from build123d import *

# Parameters (mm, degrees)
F0_W     = 127
F0_H     = 76.2
F1_DEPTH = 50.8
F2_T     = -2.54
F4_DEPTH = 76.2


with BuildPart() as f1:
    # F0 (on Top) → F1 (new body)
    with BuildSketch(Plane.XY):
        with Locations((63.5, 38.1)):
            Rectangle(F0_W, F0_H)
    extrude(amount=F1_DEPTH)

    # F2
    f2_openings = [f1.faces().sort_by_distance(p)[0] for p in [
        (63.5, 38.1, 50.8),
    ]]
    offset(amount=F2_T, openings=f2_openings)

    # F3 (on face) → F4 (join)
    with BuildSketch(Plane.XZ):
        Polygon((50.8, 50.8), (0, 0), (51.892955, 0), align=None)
    extrude(amount=F4_DEPTH)


solid = f1.part
CAD build for the part. Positions are in the model's coordinates, mm. A direction names the side the tool comes from. Coordinates: 2 decimals unless noted, no trailing zeros. Loops run counter-clockwise (first coordinate to the right, second up) from the corner with the lowest first, then second, coordinate; pieces in that order, holes last. Notation, with made-up numbers: (43, 37) - (66, 37) arc R30 ccw to (66, 70) - close; hole circle Ø5 at (72, -14.5). An arc over 180 degrees is marked (long way). Use one line per item in the form item = value. Start each with the question number.
1) Two-plate mould, pull along Y, no slides. Class faces 4 (the face through (88, 0, 25)), 5 (the face through (2.54, 38, 26)), 6 (the face through (26, -38, 26)): +Y half, -Y half, draft (parallel to the pull), parting line (faces both ways), or undercut.
2) Tool access for faces 1 (the face through (63, 2.54, 26)), 2 (the face through (14, 0, 36)), 3 (the face through (127, 38, 25)): list every direction of +Z, -Z, +X, -X, +Y, -Y with a clear straight run to the whole face (end or side of a thin tool).
3) Band-saw the part on D-D (z = 30.5). Give the cut face in (x, y), and give its area (3 significant figures).
4) Band-saw the part on A-A (x = 110.5). Give the cut face in (y, z), and give its area (3 significant figures).
5) Flat gauge pins, fed straight in: pin 1 (1 mm diameter, centred on y = 45, z = 28, fed in from -X); pin 2 (1.5 mm diameter, centred on y = -55, z = 25.5, fed in from +X); pin 3 (15 mm diameter, centred on x = 71.5, z = 21, fed in from -Y). Where does each tip first touch, or does it go through?
6) Band-saw the part on B-B (z = 20). Give the cut face in (x, y), and give its area (3 significant figures).
7) Band-saw the part on C-C (y = 11). Give the cut face in (x, z), and give its area (3 significant figures).
8) Drill centre lines: L1, parallel to Y at x = 119, z = 26.5; L2, parallel to Y at x = 44.5, z = 11; L3, parallel to X at y = 31.5, z = 33.5. Where is each one in solid material? Low to high. Write a range as from..to.
Check values:
q1.face_4 = -Y half
q1.face_5 = undercut
q1.face_6 = draft
q2.face_1 = +Z
q2.face_2 = +Z, -X, -Y
q2.face_3 = +Z, -Z, +X, +Y, -Y
q3.outline = (0, 0) - (30.5, 0) - (30.5, -76.2) - (51.24, -76.2) - (51.24, 0) - (127, 0) - (127, 76.2) - (0, 76.2) - close; hole (2.54, 2.54) - (124.46, 2.54) - (124.46, 73.66) - (2.54, 73.66) - close
q3.area = 2,590 mm2
q4.outline = (0, 0) - (76.2, 0) - (76.2, 50.8) - (73.66, 50.8) - (73.66, 2.54) - (2.54, 2.54) - (2.54, 50.8) - (0, 50.8) - close
q4.area = 439 mm2
q5.pin_1 = 0
q5.pin_2 = 51.36
q5.pin_3 = 0
q6.outline = (0, 0) - (20, 0) - (20, -76.2) - (51.46, -76.2) - (51.46, 0) - (127, 0) - (127, 76.2) - (0, 76.2) - close; hole (2.54, 2.54) - (124.46, 2.54) - (124.46, 73.66) - (2.54, 73.66) - close
q6.area = 3,400 mm2
q7.outline = (0, 0) - (127, 0) - (127, 50.8) - (124.46, 50.8) - (124.46, 2.54) - (2.54, 2.54) - (2.54, 50.8) - (0, 50.8) - close
q7.area = 568 mm2
q8.L1 = 0..2.54, 73.66..76.2
q8.L2 = -76.2..2.54, 73.66..76.2
q8.L3 = 0..2.54, 124.46..127
